Read the model definition and answer for the solid it produces. Units are mm, in the model's axes. Round coordinates to 2 decimals unless told otherwise and drop trailing zeros. Write each loop counter-clockwise with the first axis right and the second up, starting at its lowest first coordinate (ties: lowest second). Pieces come first, ordered by that corner, then holes. Notation, with made-up numbers: (35, 30) -> (84, 30) arc R17 ccw to (84, 34) -> close; hole circle Ø6 at (-14, 70.5). An arc over 180 degrees is marked (long way). Return JSON: item names as keys, results as strings. Group by question number.
(1) A cutting plane is placed at C-C on z = -11. Give the vertices of the cut face in (x, y), then the cut area to 3 significant figures.
(2) Given pin 1 (3 mm diameter, centred on x = -29.5, z = -12, fed in from -Y), flat-ended and moving along its own axis, determine where the tip first touches the part or whether it passes through.
(3) The mould has two halves that part along Z. Classify faces 1 (the flat face through (0, 2, -17.5)), 2 (the flat face through (0, 2, 17.5)), 3 (the cylindrical face through (-28.72, 2.03, -9.52)): released by +Z, released by -Z, zero draft, split by the parting line, or undercut.
(4) A cutting plane is placed at B-B on x = 29.5. Give the vertices of the cut face in (y, z), then the cut area to 3 significant figures.
(5) A cutting plane is placed at A-A on y = 1.75. Give the vertices of the cut face in (x, z), then the cut area to 3 significant figures.
(6) Straight lines are drawn through the part: line 1 (X direction, y = 1.65, z = 12); line 2 (X direction, y = 0.55, z = -12.5). For each, find the intervals that lie inside material, in ascending order.
```python
from build123d import *

# Parameters (mm, degrees)
SKETCH_1_W          = 68
SKETCH_1_H          = 35
EXTRUDE_1_DEPTH     = 4
SKETCH_2_R          = 2.6
SKETCH_2_R_2        = 2.1
CUT_EXTRUDE_1_DEPTH = 4
FILLET_1_R          = 3


with BuildPart() as part:
    # 草图1 → 凸台-拉伸1 (new body)
    with BuildSketch(Plane(origin=(0, 0, 0), x_dir=(1, 0, 0), z_dir=(0, 1, 0))):
        Rectangle(SKETCH_1_W, SKETCH_1_H)
    extrude(amount=EXTRUDE_1_DEPTH)

    # 草图2 → 切除-拉伸1 (cut)
    with BuildSketch(Plane(origin=(0, 4, 0), x_dir=(1, 0, 0), z_dir=(0, 1, 0))):
        with Locations(Location((-29.5, 12, 0), (0, 0, 270))):
            Circle(SKETCH_2_R)
        with Locations(Location((29.5, 12, 0), (0, 0, 90))):
            Circle(SKETCH_2_R)
        with Locations(Location((29.5, -12, 0), (0, 0, 270))):
            Circle(SKETCH_2_R)
        with Locations(Location((-29.5, -12, 0), (0, 0, 90))):
            Circle(SKETCH_2_R)
        with Locations(Location((0, 12, 0), (0, 0, 270))):
            Circle(SKETCH_2_R_2)
        with Locations(Location((0, -12, 0), (0, 0, 90))):
            Circle(SKETCH_2_R_2)
    extrude(amount=-CUT_EXTRUDE_1_DEPTH, mode=Mode.SUBTRACT)

    # 圆角1
    fillet_1_edges = [part.edges().sort_by_distance(p)[0] for p in [
        (34, 2, 17.5),
        (-34, 2, 17.5),
        (-34, 2, -17.5),
        (34, 2, -17.5),
    ]]
    fillet(fillet_1_edges, radius=FILLET_1_R)


solid = part.part
```
Checks:
{
 "1": {"outline": "(-34, 0) -> (-31.9, 0) -> (-31.9, 4) -> (-34, 4) -> close; (-27.1, 0) -> (-1.85, 0) -> (-1.85, 4) -> (-27.1, 4) -> close; (1.85, 0) -> (27.1, 0) -> (27.1, 4) -> (1.85, 4) -> close; (31.9, 0) -> (34, 0) -> (34, 4) -> (31.9, 4) -> close", "area": "219 mm^2"},
 "2": {"pin 1": "passes through"},
 "3": {"face 1": "released by -Z", "face 2": "released by +Z", "face 3": "undercut"},
 "4": {"outline": "(0, -17.5) -> (4, -17.5) -> (4, -14.6) -> (0, -14.6) -> close; (0, -9.4) -> (4, -9.4) -> (4, 9.4) -> (0, 9.4) -> close; (0, 14.6) -> (4, 14.6) -> (4, 17.5) -> (0, 17.5) -> close", "area": "98.4 mm^2"},
 "5": {"outline": "(-34, -14.5) arc R3 ccw to (-31, -17.5) -> (31, -17.5) arc R3 ccw to (34, -14.5) -> (34, 14.5) arc R3 ccw to (31, 17.5) -> (-31, 17.5) arc R3 ccw to (-34, 14.5) -> close; hole circle Ø5.2 at (-29.5, -12); hole circle Ø5.2 at (-29.5, 12); hole circle Ø4.2 at (0, -12); hole circle Ø4.2 at (0, 12); hole circle Ø5.2 at (29.5, -12); hole circle Ø5.2 at (29.5, 12)", "area": "2,260 mm^2"},
 "6": {"line 1": "x = -34 to -32.1, -26.9 to -2.1, 2.1 to 26.9, 32.1 to 34", "line 2": "x = -34 to -32.05, -26.95 to -2.04, 2.04 to 26.95, 32.05 to 34"}
}
